CAD build for the part. Positions are in the model's coordinates, mm. Face numbers are marked on the shaded views. A direction names the side the tool comes from. Give positions to 0.01 mm unless a question says otherwise; leave off trailing zeros. Order: outer loops, then holes, each group sorted by start corner. A loop starts at its lowest first (then second) coordinate and runs counter-clockwise, first axis right, second up.
Item 1: Band-saw the part on A-A on z = 8. Give the cut face in (x, y), plus the area to 4 significant figures.
Item 2: Which spindle directions (+Z, -Z, +X, -X, +Y, -Y) get a long thin tool onto all of the face, cutting with end or side? Do the marked faces 4, 5 and 6. Say none if no direction does.
Item 3: Band-saw the part on C-C on y = 0.5. Give the cut face in (x, z), plus the area to 3 significant figures.
Item 4: Band-saw the part on B-B on x = -4.5. Give the cut face in (y, z).
Item 5: Band-saw the part on D-D on z = 29. Give the cut face in (x, y).
Item 6: Wall check: L1, parallel to Z at x = 15, y = 0.5; L2, parallel to X at y = 18.05, z = 37; L3, parallel to X at y = 8, z = 10. Give the ranges that are in metal, low to high.
Item 7: Flat gauge pins, fed straight in: P1, Ø6, axis at x = -4.5, z = 8, coming from the -Y side; P2, Ø8, axis at y = -13, z = 37, coming from the +X side; P3, Ø5.5, axis at x = -17.5, z = 37, coming from the +Y side. Where does each tip first touch, or does it go through?
Item 8: Two-plate mould, pull along X, no slides. Class the marked faces 1, 2 and 3: released by +X, released by -X, zero draft, split by the parting line, or undercut.
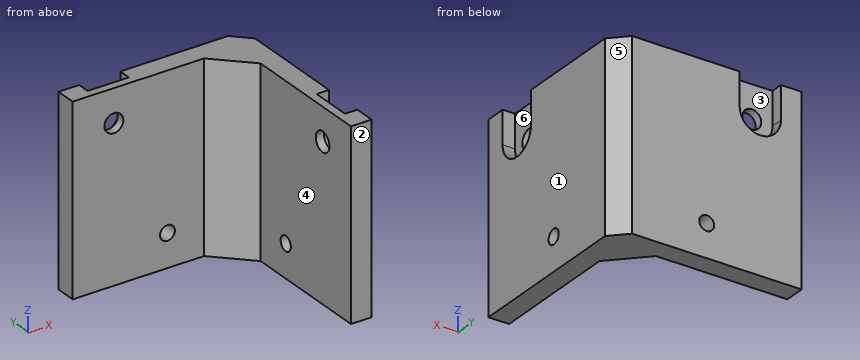
```python
from build123d import *

# Parameters (mm, degrees)
F0_W      = 45
F0_H      = 45
F1_DEPTH  = 5
F2_W      = 45
F2_H      = 5
F3_DEPTH  = 40
F5_DEPTH  = 45
F7_DEPTH  = 45.001
F9_R      = 1.8
F9_R_2    = 2.3
F10_DEPTH = 45.001
F11_R     = 2.4
F11_R_2   = 1.8
F12_DEPTH = 45.001
F13_W     = 10
F13_H     = 3
F13_W_2   = 3
F13_H_2   = 10
F14_DEPTH = 13
F15_R     = 4.99999
F16_ANGLE = -90


# Not quite as in the source:
# - a fillet or chamfer is up to 0.001 mm smaller than in the source, because OpenCascade refuses the exact size


with BuildPart() as f1:
    # F0 (on Top) → F1 (new body)
    with BuildSketch(Plane.XY):
        Rectangle(F0_W, F0_H)
    extrude(amount=F1_DEPTH)

    # F2 (on face) → F3 (join)
    with BuildSketch(Plane.XY.offset(5)):
        with Locations((0, 20)):
            Rectangle(F2_W, F2_H)
    extrude(amount=F3_DEPTH)

    # F4 (on face) → F5 (join, through all)
    with BuildSketch(Plane(origin=(-22.5, 0, 0), x_dir=(0, -1, 0), z_dir=(-1, 0, 0))):
        Polygon((-9.3682720164, 5), (-17.5, 13.1317279836), (-17.5, 5), align=None)
    extrude(amount=-F5_DEPTH)

    # F6 (on face) → F7 (cut, through all)
    with BuildSketch(Plane.YZ.offset(22.5)):
        Polygon((18.6109127035, 0), (22.5, 0), (22.5, 3.8890872965), align=None)
    extrude(amount=-F7_DEPTH, mode=Mode.SUBTRACT)

    # F9 (on face) → F10 (cut, through all)
    with BuildSketch(Plane(origin=(0, 22.5, 0), x_dir=(-1, 0, 0), z_dir=(0, 1, 0))):
        with Locations((14.5, 22)):
            Circle(F9_R)
        with Locations((-14.5, 35)):
            Circle(F9_R_2)
    extrude(amount=-F10_DEPTH, mode=Mode.SUBTRACT)

    # F11 (on face) → F12 (cut, through all)
    with BuildSketch(Plane(origin=(0, 0, 0), x_dir=(1, 0, 0), z_dir=(0, 0, -1))):
        with Locations((14.5, 12.5)):
            Circle(F11_R)
        with Locations((-14.5, -0.5)):
            Circle(F11_R_2)
    extrude(amount=-F12_DEPTH, mode=Mode.SUBTRACT)

    # F13 (on face) → F14 (cut)
    with BuildSketch(Plane.YZ.offset(22.5)):
        with Locations((-12.5, 1.5)):
            Rectangle(F13_W, F13_H)
        with Locations((21, 35)):
            Rectangle(F13_W_2, F13_H_2)
    extrude(amount=-F14_DEPTH, mode=Mode.SUBTRACT)

    # F15 (radius 5 in the source; OpenCascade refuses exactly that, so slightly less here)
    f15_edges = [f1.edges().sort_by_distance(p)[0] for p in [
        (9.5, -17.5, 1.5),
        (9.5, -7.5, 1.5),
        (9.5, 21, 30),
        (9.5, 21, 40),
    ]]
    fillet(f15_edges, radius=F15_R)


with BuildPart() as f1_1:
    # F16: moved
    add(f1.part.rotate(Axis((-22.5, -1.9445436483, 0), (0, 1, 0)), F16_ANGLE))


with BuildPart() as f1_2:
    # F17: moved
    add(f1_1.part.moved(Location((40, 0, 0))))


solid = f1_2.part
```
The answers:
1. outline: (-27.5, 17.5) - (-6.3, 17.5) - (-6.3, 22.5) - (-27.5, 22.5) - close; (-2.7, 17.5) - (4.37, 17.5) - (12.5, 9.37) - (12.5, 2.3) - (17.5, 2.3) - (17.5, 18.61) - (13.61, 22.5) - (-2.7, 22.5) - close; (12.5, -22.5) - (17.5, -22.5) - (17.5, -1.3) - (12.5, -1.3) - close
1. area: 414.5 mm2
2. face 4: +Z, -Z, -X, -Y
2. face 5: +Z, -Z, +X, +Y
2. face 6: +Z, +X
3. outline: (12.5, 0) - (17.5, 0) - (17.5, 6.2) - (12.5, 6.2) - close; (12.5, 9.8) - (17.5, 9.8) - (17.5, 45) - (12.5, 45) - close
3. area: 207 mm2
4. outline: (17.5, 0) - (22.5, 0) - (22.5, 6.2) - (17.5, 6.2) - close; (17.5, 9.8) - (22.5, 9.8) - (22.5, 45) - (17.5, 45) - close
5. outline: (-27.5, 17.5) - (4.37, 17.5) - (12.5, 9.37) - (12.5, -22.5) - (17.5, -22.5) - (17.5, 18.61) - (13.61, 22.5) - (-27.5, 22.5) - close
6. L1: z = 0 to 6.2, 9.8 to 45
6. L2: x = -27.5 to -19.8, -15.2 to 17.5
6. L3: x = 12.5 to 17.5
7. P1: stops at y = 17.5
7. P2: stops at x = 14.5
7. P3: stops at y = 19.5
8. face 1: released by +X
8. face 2: zero draft
8. face 3: undercut
